Part model, mm, in its own coordinate system. A direction names the side the tool comes from. Round coordinates to 2 decimals unless told otherwise and drop trailing zeros. Loops run counter-clockwise (first coordinate to the right, second up) from the corner with the lowest first, then second, coordinate; pieces in that order, holes last.
1) Band-saw the part on D-D, the plane x = 99. Write the cut outline in (y, z), then the cut area to 3 significant figures.
2) Band-saw the part on B-B, the plane y = 10. Write the cut outline in (x, z).
3) Band-saw the part on A-A, the plane z = 66. Write the cut outline in (x, y) (3 decimals).
4) Band-saw the part on C-C, the plane x = -97.5. Write the cut outline in (y, z), then the cut area to 3 significant figures.
5) Probe line 1 (X direction, y = 27.5, z = -24.5); line 2 (Z direction, x = 137.5, y = 6.5); line 3 (Y direction, x = -125, z = -98.8). List the from-to ranges inside material, lowest first.
6) Mould opens along X. For faces 1 (the cylindrical face through (-117.37, 12.4, 97.54)), 2 (the flat face through (175, 25, 1)), 3 (the flat face through (-2, 0, -1)) say: +X half, -X half, draft (parallel to the pull), parting line (faces both ways), or undercut.
7) 3-axis set-ups, long thin cutter, end or side, ignore diameter. For faces 4 (the flat face through (-1, 50, -97)), 5 (the flat face through (2, 25, -95)): which of +Z, -Z, +X, -X, +Y, -Y reach the whole face in a straight line?
8) Drop flat-ended pins along their axis: P1, Ø1.5, axis at x = 72, z = 60.5, coming from the +Y side; P2, Ø9.5, axis at x = 125, y = 10, coming from the -Z side (3 decimals). Give the stop position or say it passes through.
from build123d import *

# Parameters (mm, degrees)
SKETCH1_W           = 350
SKETCH1_H           = 200
BOSS_EXTRUDE1_DEPTH = 50
SHELL1_T            = -5
CUT_EXTRUDE1_REACH  = 272.416
SKETCH3_R           = 8
SKETCH4_W           = 17.489995996
SKETCH4_H           = 190
SKETCH4_W_2         = 5
CUT_EXTRUDE4_DEPTH  = 10
SKETCH5_W           = 102.489995996
SKETCH5_H           = 30
CUT_EXTRUDE5_DEPTH  = 10


with BuildPart() as part:
    # Sketch1 → Boss-Extrude1 (new body)
    with BuildSketch(Plane(origin=(0, 0, 0), x_dir=(1, 0, 0), z_dir=(0, 1, 0))):
        Rectangle(SKETCH1_W, SKETCH1_H)
    extrude(amount=BOSS_EXTRUDE1_DEPTH)

    # Shell1
    shell1_openings = [part.faces().sort_by_distance(p)[0] for p in [
        (0, 50, 0),
    ]]
    offset(amount=SHELL1_T, openings=shell1_openings, kind=Kind.INTERSECTION)

    # Cut-Extrude1: up to this face of the body (flat: up to its plane)
    cut_extrude1_end = Plane(part.part.faces().sort_by_distance((0, 25, -100))[0])
    # Sketch3 → Cut-Extrude1 (cut, up to the picked face)
    with BuildSketch(Plane.XY.offset(100), mode=Mode.PRIVATE) as cut_extrude1_sk1:
        with Locations((-125, 10)):
            Circle(SKETCH3_R)
    cut_extrude1_tool1 = split(extrude(cut_extrude1_sk1.sketch, amount=-CUT_EXTRUDE1_REACH, mode=Mode.PRIVATE), bisect_by=cut_extrude1_end, keep=Keep.BOTH, mode=Mode.PRIVATE)
    # Sketch3 → Cut-Extrude1 (cut, up to the picked face)
    with BuildSketch(Plane.XY.offset(100), mode=Mode.PRIVATE) as cut_extrude1_sk2:
        with Locations((125, 10)):
            Circle(SKETCH3_R)
    cut_extrude1_tool2 = split(extrude(cut_extrude1_sk2.sketch, amount=-CUT_EXTRUDE1_REACH, mode=Mode.PRIVATE), bisect_by=cut_extrude1_end, keep=Keep.BOTH, mode=Mode.PRIVATE)
    add(cut_extrude1_tool1.solids().sort_by(Axis((-125, 10, 100), (0, 0, -1)))[0], mode=Mode.SUBTRACT)
    add(cut_extrude1_tool2.solids().sort_by(Axis((125, 10, 100), (0, 0, -1)))[0], mode=Mode.SUBTRACT)

    # Sketch4 → Cut-Extrude4 (cut)
    with BuildSketch(Plane(origin=(0, 5, 0), x_dir=(1, 0, 0), z_dir=(0, 1, 0))):
        with Locations((-127.5, 0)):
            Rectangle(SKETCH4_W, SKETCH4_H)
        with Locations((-116.255002002, 0)):
            Rectangle(SKETCH4_W_2, SKETCH4_H)
        with Locations((116.255002002, 0)):
            Rectangle(SKETCH4_W_2, SKETCH4_H)
        with Locations((127.5, 0)):
            Rectangle(SKETCH4_W, SKETCH4_H)
    extrude(amount=-CUT_EXTRUDE4_DEPTH, mode=Mode.SUBTRACT)

    # Sketch5 → Cut-Extrude5 (cut)
    with BuildSketch(Plane(origin=(0, 5, 0), x_dir=(1, 0, 0), z_dir=(0, 1, 0))):
        with Locations((-105, 0)):
            Rectangle(SKETCH5_W, SKETCH5_H)
    extrude(amount=-CUT_EXTRUDE5_DEPTH, mode=Mode.SUBTRACT)


solid = part.part
Reported:
1. outline: (0, -100) - (50, -100) - (50, -95) - (5, -95) - (5, 95) - (50, 95) - (50, 100) - (0, 100) - close
1. area: 1,450 mm2
2. outline: (-175, -100) - (-133, -100) - (-133, -95) - (-170, -95) - (-170, 95) - (-133, 95) - (-133, 100) - (-175, 100) - close; (-117, -100) - (117, -100) - (117, -95) - (-117, -95) - close; (-117, 95) - (117, 95) - (117, 100) - (-117, 100) - close; (133, -100) - (175, -100) - (175, 100) - (133, 100) - (133, 95) - (170, 95) - (170, -95) - (133, -95) - close
3. outline: (-175, 0) - (-136.245, 0) - (-136.245, 5) - (-170, 5) - (-170, 50) - (-175, 50) - close; (-113.755, 0) - (113.755, 0) - (113.755, 5) - (-113.755, 5) - close; (136.245, 0) - (175, 0) - (175, 50) - (170, 50) - (170, 5) - (136.245, 5) - close
4. outline: (0, -100) - (50, -100) - (50, -95) - (5, -95) - (5, -15) - (0, -15) - close; (0, 15) - (5, 15) - (5, 95) - (50, 95) - (50, 100) - (0, 100) - close
4. area: 1,300 mm2
5. line 1: x = -175 to -170, 170 to 175
5. line 2: z = -100 to -95, 95 to 100
5. line 3: y = 0 to 2, 18 to 50
6. face 1: undercut
6. face 2: +X half
6. face 3: draft
7. face 4: +Z, -Z, +X, -X, +Y
7. face 5: +Y
8. P1: stops at y = 5
8. P2: passes through
